```python
from build123d import *


with BuildPart() as part:
    # 草图1 → 旋转1 (revolve)
    with BuildSketch(Plane.XY, mode=Mode.PRIVATE) as revolve_1_sk:
        with BuildLine():
            Line((0, -8.871116041), (-4.6, -8.871116041))
            Line((-4.6, -8.871116041), (-3.9, 66.878718358))
            Line((-3.9, 66.878718358), (-2.9, 66.878718358))
            Line((-2.9, 66.878718358), (-2.9, 67.678718358))
            Line((-2.9, 67.678718358), (-3.9, 67.678718358))
            Line((-3.9, 67.678718358), (-3.9, 68.478718358))
            Line((-3.9, 68.478718358), (-2.9, 68.478718358))
            Line((-2.9, 68.478718358), (-2.9, 69.316506289))
            Line((-2.9, 69.316506289), (-3.735091076, 69.316506289))
            Line((-3.735091076, 69.316506289), (-3.735091076, 75.816506289))
            ThreePointArc((-3.735091076, 75.816506289), (-2.337753917, 77.847174239), (0, 78.628883959))
            Line((0, 78.628883959), (0, -8.871116041))
        make_face()
    revolve(revolve_1_sk.sketch.rotate(Axis((0, 100.774977187, 0), (0, -1, 0)), 270), axis=Axis((0, 100.774977187, 0), (0, -1, 0)))

    # 草图2 → Revolve 883 (revolve)
    with BuildSketch(Plane(origin=(0, 0, 0), x_dir=(0, 0, -1), z_dir=(1, 0, 0)), mode=Mode.PRIVATE) as revolve_883_sk:
        Polygon((0, 0), (-6.429276603, 0), (-6.429276603, 1.099364131), (-12.95, 1.099364131), (-12.95, -0.266872358), (-14.47347065, -0.266872358), (-14.47347065, 1.099364131), (-17.7, 1.099364131), (-17.7, 2.489950524), (-25.109397803, 2.489950524), (-25.109397803, 2.389950524), (-25.9, 2.389950524), (-25.9, -2.510049476), (0, -2.510049476), align=None)
    revolve(revolve_883_sk.sketch.rotate(Axis((0, -2.510049476, 44.503458482), (0, 0, -1)), 90), axis=Axis((0, -2.510049476, 44.503458482), (0, 0, -1)))


solid = part.part
```
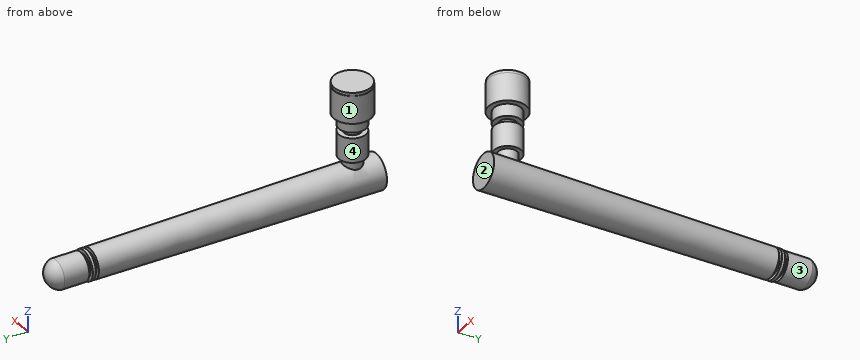
Can you work these out from the model? Positions are in its coordinate system, mm. Face numbers are marked on the shaded views. A direction names the side the tool comes from. Coordinates: 2 decimals unless noted, no trailing zeros. Write each loop counter-clockwise with the first axis right and the second up, starting at its lowest first coordinate (ties: lowest second). Pieces come first, ordered by that corner, then holes. Notation, with made-up numbers: M 45,61.25 L 68,61.25 A17 ccw 68,83.25 Z; hole C 68.25,0 d7. An arc over 180 degrees is marked long. Write item = value, one per line. Start each with the question number.
Q1. If I drill on L1, parallel to Y at x = 1.5, z = 3; L2, parallel to Y at x = -1.75, z = -2.5; L3, parallel to Y at x = 1.25, z = 23, over which ranges is the centre line in solid material (lowest first)? Write a range as [from, to].
Q2. On a 3-axis mill with a long thin cutter (end or side, diameter ignored), from which of +Z, -Z, +X, -X, +Y, -Y can I reach the whole of each face in a straight line? I mean the marked faces 1, 2, 3 and 4. Say none if no direction works.
Q3. I'm going to push flat-ended pins straight in: pin 1 (2 mm diameter, centred on x = 2.5, y = 10.5, fed in from +Z); pin 2 (5 mm diameter, centred on y = 60, z = -1.5, fed in from +X); pin 3 (5 mm diameter, centred on x = -1.5, y = -4.5, fed in from -Z); pin 4 (1.5 mm diameter, centred on y = 36, z = 6, fed in from +X). Where does each tip first touch, or does it pass through?
Q4. If we section it at A-A, the plane z = 16.5: Write out the boundary of the cut face in (x, y), then the cut area to 3 significant figures.
Q5. If we section it at B-B, the plane y = 70.5: Write out the boundary of the cut face in (x, z).
Check sheet entries:
q1.L1 = [-8.87, 66.88], [67.68, 68.48], [69.32, 76.71]
q1.L2 = [-8.87, 66.88], [67.68, 68.48], [69.32, 77.15]
q1.L3 = [-7.35, 2.33]
q2.face_1 = +Z
q2.face_2 = +Z, -Z, +X, -X, -Y
q2.face_3 = +Y
q2.face_4 = none
q3.pin_1 = 4.16
q3.pin_2 = 3.98
q3.pin_3 = -4.58
q3.pin_4 = through
q4.outline = C 0,-2.51 d7.22
q4.area = 40.9 mm²
q5.outline = C 0,0 d7.47
